The model under review builds one solid part; all positions refer to its coordinate system, in mm. Face numbers are marked on the shaded views. A direction names the side the tool comes from. Give positions to 0.01 mm unless a question says otherwise; leave off trailing zeros. Loops run counter-clockwise (first coordinate to the right, second up) from the corner with the lowest first, then second, coordinate; pieces in that order, holes last. Notation, with made-up numbers: M 80.25,55.5 L 110.25,55.5 A21 ccw 110.25,82.5 Z; hole C -17,52 d3. An arc over 180 degrees is marked long. Write item = value, one per line. Start each with the question number.
1. We need section A-A on x = 38.5. Give the boundary of the cut face in (y, z) (1 decimal), then the cut area to 3 significant figures.
2. Draft analysis for pull direction Z (two halves, no side actions). For the marked faces 1, 2, 3 and 4, state which applies: pulls with the +Z half, pulls with the -Z half, needs draft (parallel to the pull), parting line crosses it, or undercut.
3. Wall thickness on line 1 along Y through (x, z) = (4, 0); line 2 along Y through (x, z) = (40.25, 0); line 3 along Z through (x, y) = (6, 33.5): over which ranges is each line inside the solid? List them lowest first. Write a range as from..to.
4. For pin 1 (13 mm diameter, centred on y = -3, z = 0.5, fed in from +X) (3 decimals); pin 2 (1.8 mm diameter, centred on y = 0, z = 33.34, fed in from -X); pin 3 (3 mm diameter, centred on y = 13.36, z = -49.87, fed in from +X) (3 decimals); pin 4 (2.5 mm diameter, centred on y = -25.81, z = 44.71, fed in from +X), all flat-tipped, find the tip position at first contact; note any pin that passes through.
5. For the marked faces 5, 6 and 7, list the 3-axis set-ups (+Z, -Z, +X, -X, +Y, -Y) from which the entire face can be reached by the end or side of a thin tool; tool diameter is ignored.
6. We need section B-B on x = 27. Give the boundary of the cut face in (y, z).
from build123d import *

# Parameters (mm, degrees)
SKETCH3_R                       = 4.7625
OXIDIZER_INLET_HOLE_DEPTH       = 93.199999203
FLANGE_HOLES_D                  = 2.8702
DOWEL_HOLES_D                   = 4.7625
DOWEL_HOLES_DEPTH               = 6.35
DOWEL_HOLES_TIP                 = 1.430799349
SKETCH12_R                      = 38.1
IMPINGING_PLATE_FLAT_CUT_DEPTH  = 3.81
SKETCH14_R                      = 38.1
SKETCH15_R                      = 38.1
SKETCH16_R                      = 28.575
SKETCH17_R                      = 4.7625
SKETCH21_R                      = 28.575
CUT_EXTRUDE1_DEPTH              = 9.525
INTERNAL_FILLET_R               = 3.175
EXTENDED_8_BC_COUNT             = 8
CHAMFER_FOR_IMPINGING_EDGE_SIZE = 0.127


with BuildPart() as part:
    # Sketch2 → Main Structure (revolve)
    with BuildSketch(Plane.XY, mode=Mode.PRIVATE) as main_structure_sk:
        Polygon((0, 0), (0, 56.35625), (9.525, 56.35625), (9.525, 45.72), (19.05, 45.72), (31.75, 13.081), (44.45, 13.081), (44.45, 6.2484), (46.355, 6.2484), (46.355, 0), align=None)
    revolve(main_structure_sk.sketch.rotate(Axis((0, 0, 0), (1, 0, 0)), 90), axis=Axis((0, 0, 0), (1, 0, 0)))

    # Sketch3 → Oxidizer Inlet Hole (cut, through all)
    with BuildSketch(Plane(origin=(46.355, 0, 0), x_dir=(0, 0, -1), z_dir=(1, 0, 0))):
        Circle(SKETCH3_R)
    extrude(amount=-OXIDIZER_INLET_HOLE_DEPTH, mode=Mode.SUBTRACT)

    # Flange Holes (through all)
    with Locations(Plane.ZY):
        with Locations((0, -51.6255), (-25.81275, -44.708994483), (-44.708994483, -25.81275), (-51.6255, 0), (-44.708994483, 25.81275), (-25.81275, 44.708994483), (0, 51.6255), (25.81275, 44.708994483), (44.708994483, 25.81275), (51.6255, 0), (44.708994483, -25.81275), (25.81275, -44.708994483)):
            Hole(FLANGE_HOLES_D / 2)

    # Dowel Holes
    with Locations(Plane.ZY):
        with Locations((49.866403745, -13.361662613), (-49.866403745, 13.361662613)):
            Hole(DOWEL_HOLES_D / 2, depth=DOWEL_HOLES_DEPTH)
            with Locations((0, 0, -(DOWEL_HOLES_DEPTH + DOWEL_HOLES_TIP / 2))):  # 118° drill point
                Cone(0, DOWEL_HOLES_D / 2, DOWEL_HOLES_TIP, mode=Mode.SUBTRACT)

    # Sketch12 → Impinging Plate Flat Cut (cut)
    with BuildSketch(Plane.ZY):
        Circle(SKETCH12_R)
    extrude(amount=-IMPINGING_PLATE_FLAT_CUT_DEPTH, mode=Mode.SUBTRACT)

    # Sketch14 → Impinging Plate Taper Cut section 0
    with BuildSketch(Plane.ZY.offset(-3.81)):
        Circle(SKETCH14_R)
    # Sketch15 → Impinging Plate Taper Cut section 1
    with BuildSketch(Plane.ZY.offset(-6.35)):
        Circle(SKETCH15_R)
    loft(mode=Mode.SUBTRACT)

    # Sketch16 → Internal Flow Path Loft Cut section 0
    with BuildSketch(Plane.ZY.offset(-15.875)):
        Circle(SKETCH16_R)
    # Sketch17 → Internal Flow Path Loft Cut section 1
    with BuildSketch(Plane.ZY.offset(-31.115)):
        Circle(SKETCH17_R)
    loft(mode=Mode.SUBTRACT)

    # Sketch21 → Cut-Extrude1 (cut)
    with BuildSketch(Plane.ZY.offset(-6.35)):
        Circle(SKETCH21_R)
    extrude(amount=-CUT_EXTRUDE1_DEPTH, mode=Mode.SUBTRACT)

    # Internal Fillet
    internal_fillet_edges = [part.edges().sort_by_distance(p)[0] for p in [
        (31.115, 4.7625, 0),
    ]]
    fillet(internal_fillet_edges, radius=INTERNAL_FILLET_R)

    # Sketch20 → 4-40 Tapped Holes (revolve, cut)
    with BuildSketch(Plane(origin=(6.35, 0, 33.3375), x_dir=(0, 0, 1), z_dir=(0, 1, 0))):
        Polygon((0, 0), (0, 3.854152758), (1.1303, 3.175), (1.1303, 0), align=None)
    f_4_40_tapped_holes = revolve(axis=Axis((0, 0, 33.3375), (1, 0, 0)), mode=Mode.SUBTRACT)

    # Extended 8 BC: 4-40 Tapped Holes ×8 about axis
    extended_8_bc_axis = Axis((0, 0, 0), (1, 0, 0))
    for i in range(1, EXTENDED_8_BC_COUNT):
        add(f_4_40_tapped_holes.rotate(extended_8_bc_axis, i * 360 / EXTENDED_8_BC_COUNT), mode=Mode.SUBTRACT)

    # Chamfer for Impinging Edge
    chamfer_for_impinging_edge_edges = [part.edges().sort_by_distance(p)[0] for p in [
        (6.35, 0, -38.1),
    ]]
    chamfer(chamfer_for_impinging_edge_edges, length=CHAMFER_FOR_IMPINGING_EDGE_SIZE)


solid = part.part
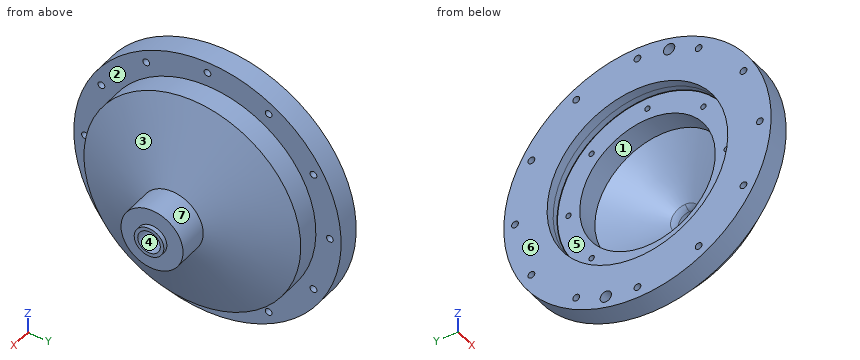
Final values:
q1.outline = C 0,0 d26.2; hole C 0,0 d9.5
q1.area = 466 mm²
q2.face_1 = undercut
q2.face_2 = needs draft
q2.face_3 = parting line crosses it
q2.face_4 = undercut
q3.line_1 = -56.36..-53.06, -50.19..-38.1, 38.1..50.19, 53.06..56.36
q3.line_2 = -13.08..-4.76, 4.76..13.08
q3.line_3 = -45.32..-18.15, 18.15..45.32
q4.pin_1 = 46.355
q4.pin_2 = 9.66
q4.pin_3 = 9.525
q4.pin_4 = through
q5.face_5 = -X
q5.face_6 = +Z, -Z, -X, +Y, -Y
q5.face_7 = +X
q6.outline = C 0,0 d50.58; hole C 0,0 d22.38
